Can you work these out from the drawing? Everything is in mm from the part's minimum corner. A direction names the side the tool comes from. Coordinates: 2 decimals unless noted, no trailing zeros. Order: outer loops, then holes, each group sorted by start corner. A loop starts at its lowest first (then second) coordinate and runs counter-clockwise, first axis right, second up. Notation, with made-up numbers: M 14,21.5 L 66,21.5 A17 ccw 66,28.5 Z; hole C 29.5,-23 d9. An arc over 180 degrees is marked long. Answer as a JSON object with one key per item and string values.
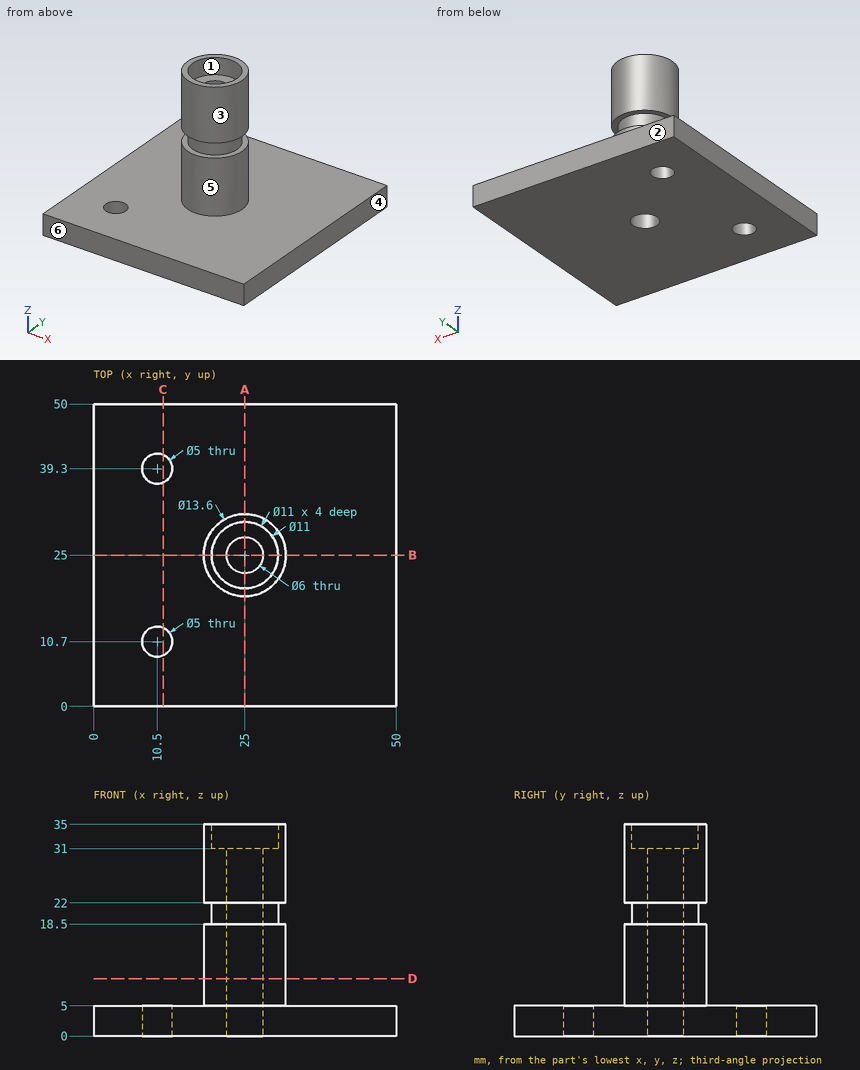
Item 1: I'm going to push flat-ended pins straight in: pin 1 (4.5 mm diameter, centred on x = 10.5, y = 10.7, fed in from -Z); pin 2 (7 mm diameter, centred on x = 25, y = 25, fed in from -Z); pin 3 (6.5 mm diameter, centred on x = 25, y = 25, fed in from +Z); pin 4 (8 mm diameter, centred on y = 35, z = 24, fed in from +X). Where does each tip first touch, or does it pass through?
Answers follow:
{"pin 1": "passes through", "pin 2": "stops at z = 0", "pin 3": "stops at z = 31", "pin 4": "stops at x = 28.2"}
Item 2: I want a section at D-D, the plane z = 9.5. Write out the boundary of the cut face in (x, y).
Answers follow:
{"outline": "C 25,25 d13.6; hole C 25,25 d6"}
Item 3: Please list where these lines run through material, in increasing order: line 1 (Y direction, x = 25, z = 32); line 2 (Y direction, x = 25, z = 9.5); line 3 (Z direction, x = 23, y = 8).
Answers follow:
{"line 1": "y = 18.2 to 19.5, 30.5 to 31.8", "line 2": "y = 18.2 to 22, 28 to 31.8", "line 3": "z = 0 to 5"}
Item 4: If we mould it in two halves opening along Y, with no side actions, what happens to the marked faces 1, 2, 3 and 4? For each: pulls with the +Y half, pulls with the -Y half, needs draft (parallel to the pull), parting line crosses it, or undercut.
Answers follow:
{"face 1": "undercut", "face 2": "pulls with the +Y half", "face 3": "parting line crosses it", "face 4": "needs draft"}
Item 5: I want a section at A-A, the plane x = 25. Write out the boundary of the cut face in (y, z).
Answers follow:
{"outline": "M 0,0 L 22,0 L 22,31 L 19.5,31 L 19.5,35 L 18.2,35 L 18.2,22 L 19.5,22 L 19.5,18.5 L 18.2,18.5 L 18.2,5 L 0,5 Z; M 28,0 L 50,0 L 50,5 L 31.8,5 L 31.8,18.5 L 30.5,18.5 L 30.5,22 L 31.8,22 L 31.8,35 L 30.5,35 L 30.5,31 L 28,31 Z"}
Item 6: Which directions (+Z, -Z, +X, -X, +Y, -Y) give clear straight access to the entire face, cutting with the end or side of a thin tool? Please do the marked faces 5 and 6.
Answers follow:
{"face 5": "+Z", "face 6": "+Z, -Z, +X, -X, -Y"}
Item 7: I want a section at C-C, the plane x = 11.5. Write out the boundary of the cut face in (y, z), plus the area to 3 significant figures.
Answers follow:
{"outline": "M 0,0 L 8.41,0 L 8.41,5 L 0,5 Z; M 12.99,0 L 37.01,0 L 37.01,5 L 12.99,5 Z; M 41.59,0 L 50,0 L 50,5 L 41.59,5 Z", "area": "204 mm^2"}
